Answer from the drawing. Dimensions are ordinates in mm from the lowest x, y and z of the part. A direction names the side the tool comes from. Coordinates: 2 decimals unless noted, no trailing zeros. Loops run counter-clockwise (first coordinate to the right, second up) from the corner with the lowest first, then second, coordinate; pieces in that order, holes last. Notation, with made-up numbers: (42.25, -11) - (46.25, -11) arc R27 cw to (46.25, 14) - close; hole circle Ø7 at (-8.75, -26.5). An arc over 180 degrees is marked (long way). Use one line per item in the form item = value. Start each with the question number.
1) A cutting plane is placed at B-B (y = 18). Give the vertices of the cut face in (x, z).
2) Consider line 1 (Z direction, x = 11, y = 18); line 2 (Y direction, x = 12.25, z = 18.25); line 3 (Y direction, x = 7.75, z = 5.25). Determine where each line is inside the solid, lowest interval first.
3) A cutting plane is placed at D-D (y = 42). Give the vertices of the cut face in (x, z), and give its area (3 significant figures).
4) A cutting plane is placed at C-C (z = 8.75). Give the vertices of the cut face in (x, y).
5) A cutting plane is placed at A-A (x = 9.75). Give the vertices of the cut face in (y, z).
6) This flat-tipped pin is pushed along its axis until it touches: P1, Ø1.5, axis at y = 35, z = 19.5, coming from the -X side. Where does it stop, or does it pass through?
7) Which of the six approach directions +Z, -Z, +X, -X, +Y, -Y give full straight-line access (tool end or side, diameter ignored) to the marked faces 1 and 2?
8) The mould has two halves that part along Y. Classify the marked faces 3, 4 and 5: released by +Y, released by -Y, zero draft, split by the parting line, or undercut.
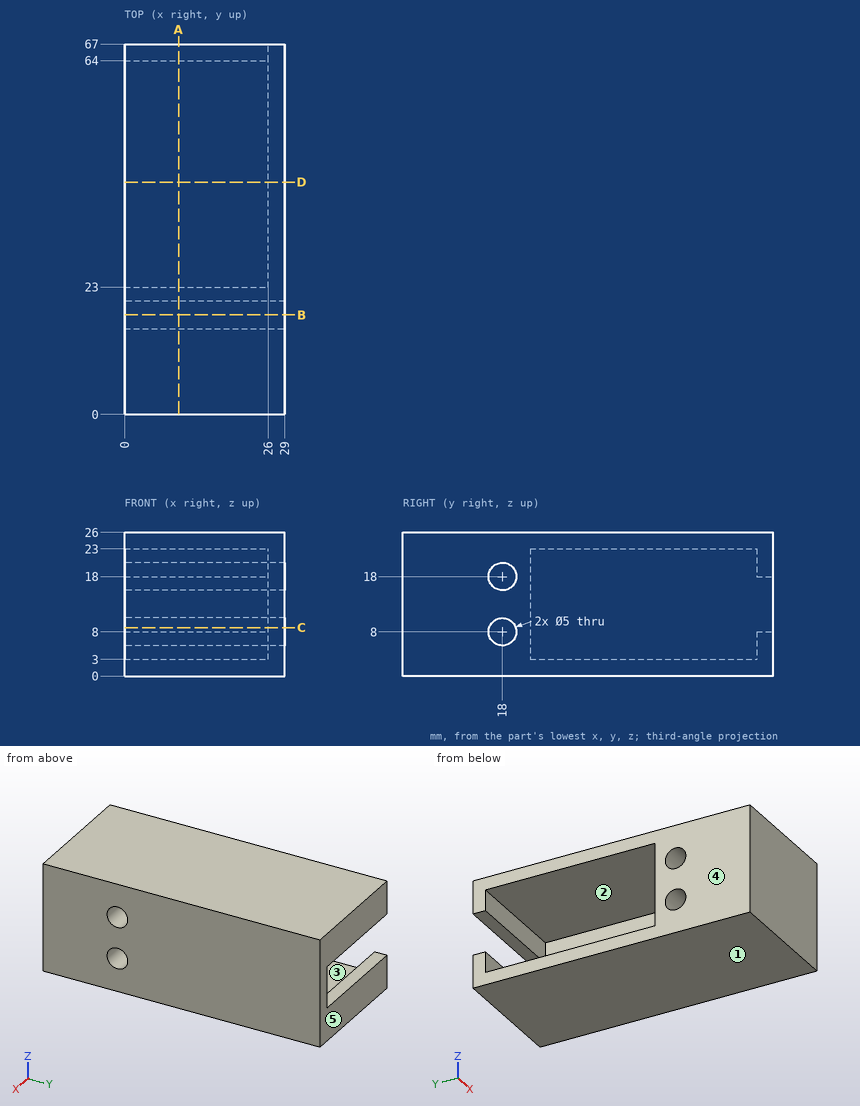
Found:
q1.outline = (0, 0) - (29, 0) - (29, 5.5) - (0, 5.5) - close; (0, 10.5) - (29, 10.5) - (29, 15.5) - (0, 15.5) - close; (0, 20.5) - (29, 20.5) - (29, 26) - (0, 26) - close
q2.line_1 = 0 to 5.5, 10.5 to 15.5, 20.5 to 26
q2.line_2 = 0 to 15.51, 20.49 to 23, 64 to 67
q2.line_3 = 0 to 23, 64 to 67
q3.outline = (0, 0) - (29, 0) - (29, 26) - (0, 26) - (0, 23) - (26, 23) - (26, 3) - (0, 3) - close
q3.area = 234 mm^2
q4.outline = (0, 0) - (29, 0) - (29, 15.62) - (0, 15.62) - close; (0, 20.38) - (29, 20.38) - (29, 67) - (26, 67) - (26, 23) - (0, 23) - close
q5.outline = (0, 0) - (67, 0) - (67, 8) - (64, 8) - (64, 3) - (23, 3) - (23, 23) - (64, 23) - (64, 18) - (67, 18) - (67, 26) - (0, 26) - close; hole circle Ø5 at (18, 8); hole circle Ø5 at (18, 18)
q6.P1 = 26
q7.face_1 = -Z, +X, -X, +Y, -Y
q7.face_2 = -X
q8.face_3 = undercut
q8.face_4 = zero draft
q8.face_5 = released by +Y
